Verification items for the finished model (mm, model axes). A direction names the side the tool comes from. Coordinates: 2 decimals unless noted, no trailing zeros. Order: outer loops, then holes, each group sorted by start corner. A loop starts at its lowest first (then second) coordinate and runs counter-clockwise, first axis right, second up. Notation, with made-up numbers: M 42,-17 L 57,-17 A10 ccw 57,-2 Z; hole C -16.75,87 d8. An arc over 180 degrees is marked long. Return JSON: item names as keys, results as strings. Group by question number.
1. Section check B-B, the plane y = 12. Record the cut outline in (x, z), plus the area to 3 significant figures.
2. Gauge pin test, flat ends, axial feed: pin 1 (1.5 mm diameter, centred on y = -7.5, z = 1.5, fed in from +X); pin 2 (1.5 mm diameter, centred on y = 1, z = 2, fed in from -X). Record the tip position at first contact, or that the pin passes through.
3. Section check C-C, the plane z = 2.15. Record the cut outline in (x, y).
4. Section check A-A, the plane x = 24. Record the cut outline in (y, z), plus the area to 3 significant figures.
5. Material ranges on line 1 along X through (y, z) = (-1, 0.85); line 2 along Y through (x, z) = (26.5, 0.45); line 3 along X through (y, z) = (8.5, 1.05), recorded low to high.
6. Mould release check, pull along X, two halves, no side actions. Record for faces 1 (the cylindrical face through (31.93, 0.35, 2.4)), 2 (the cylindrical face through (-16.7, 16.3, 2.6)), 3 (the flat face through (0, 0, 3)): +X half, -X half, draft (parallel to the pull), parting line (faces both ways), or undercut.
7. Set-up check for faces 4 (the flat face through (-7.5, 12, 1)), 5 (the flat face through (0, 0, 0)), 6 (the cylindrical face through (28.3, -1.2, 2.6)): record each of +Z, -Z, +X, -X, +Y, -Y from which the full face is reachable in a straight line by a thin tool's end or side.
```python
from build123d import *

# Parameters (mm, degrees)
F0_W     = 65
F0_H     = 50
F0_W_2   = 10
F0_H_2   = 2.5
F0_W_3   = 15
F0_H_3   = 15
F1_DEPTH = 3
F2_R     = 2


with BuildPart() as f1:
    # F0 (on Top) → F1 (new body)
    with BuildSketch(Plane.XY):
        Rectangle(F0_W, F0_H)
        with Locations((-22.5, -1.25)):
            Rectangle(F0_W_2, F0_H_2, mode=Mode.SUBTRACT)
        with Locations((22.5, -1.25)):
            Rectangle(F0_W_2, F0_H_2, mode=Mode.SUBTRACT)
        with Locations((-22.5, 16.25)):
            Rectangle(F0_W_2, F0_H_2, mode=Mode.SUBTRACT)
        with Locations((0, 12.5)):
            Rectangle(F0_W_3, F0_H_3, mode=Mode.SUBTRACT)
        with Locations((22.5, 16.25)):
            Rectangle(F0_W_2, F0_H_2, mode=Mode.SUBTRACT)
    extrude(amount=F1_DEPTH)

    # F2
    f2_edges = [f1.edges().sort_by_distance(p)[0] for p in [
        (-22.5, 17.5, 3),
        (-22.5, 15, 3),
        (-27.5, 16.25, 3),
        (-17.5, 16.25, 3),
        (0, 25, 3),
        (-32.5, 0, 3),
        (-22.5, -2.5, 3),
        (0, -25, 3),
        (-22.5, 0, 3),
        (-27.5, -1.25, 3),
        (-17.5, -1.25, 3),
        (22.5, 15, 3),
        (22.5, 17.5, 3),
        (17.5, 16.25, 3),
        (27.5, 16.25, 3),
        (32.5, 0, 3),
        (22.5, 0, 3),
        (17.5, -1.25, 3),
        (22.5, -2.5, 3),
        (27.5, -1.25, 3),
    ]]
    fillet(f2_edges, radius=F2_R)


solid = f1.part
```
Answers follow:
{
 "1": {"outline": "M -32.5,0 L -7.5,0 L -7.5,3 L -30.5,3 A2 ccw -32.5,1 Z; M 7.5,0 L 32.5,0 L 32.5,1 A2 ccw 30.5,3 L 7.5,3 Z", "area": "148 mm^2"},
 "2": {"pin 1": "x = 32.5", "pin 2": "x = -32.48"},
 "3": {"outline": "M -32.14,-24.64 L 32.14,-24.64 L 32.14,24.64 L -32.14,24.64 Z; hole M -27.86,-2.86 L -17.14,-2.86 L -17.14,0.36 L -27.86,0.36 Z; hole M -27.86,14.64 L -17.14,14.64 L -17.14,17.86 L -27.86,17.86 Z; hole M -7.5,5 L 7.5,5 L 7.5,20 L -7.5,20 Z; hole M 17.14,-2.86 L 27.86,-2.86 L 27.86,0.36 L 17.14,0.36 Z; hole M 17.14,14.64 L 27.86,14.64 L 27.86,17.86 L 17.14,17.86 Z"},
 "4": {"outline": "M -25,0 L -2.5,0 L -2.5,1 A2 ccw -4.5,3 L -23,3 A2 ccw -25,1 Z; M 0,0 L 15,0 L 15,1 A2 ccw 13,3 L 2,3 A2 ccw 0,1 Z; M 17.5,0 L 25,0 L 25,1 A2 ccw 23,3 L 19.5,3 A2 ccw 17.5,1 Z", "area": "130 mm^2"},
 "5": {"line 1": "-32.5 to -27.5, -17.5 to 17.5, 27.5 to 32.5", "line 2": "-25 to -2.5, 0 to 15, 17.5 to 25", "line 3": "-32.5 to -7.5, 7.5 to 32.5"},
 "6": {"face 1": "+X half", "face 2": "undercut", "face 3": "draft"},
 "7": {"face 4": "+Z, -Z", "face 5": "-Z, +X, -X, +Y, -Y", "face 6": "+Z"}
}
